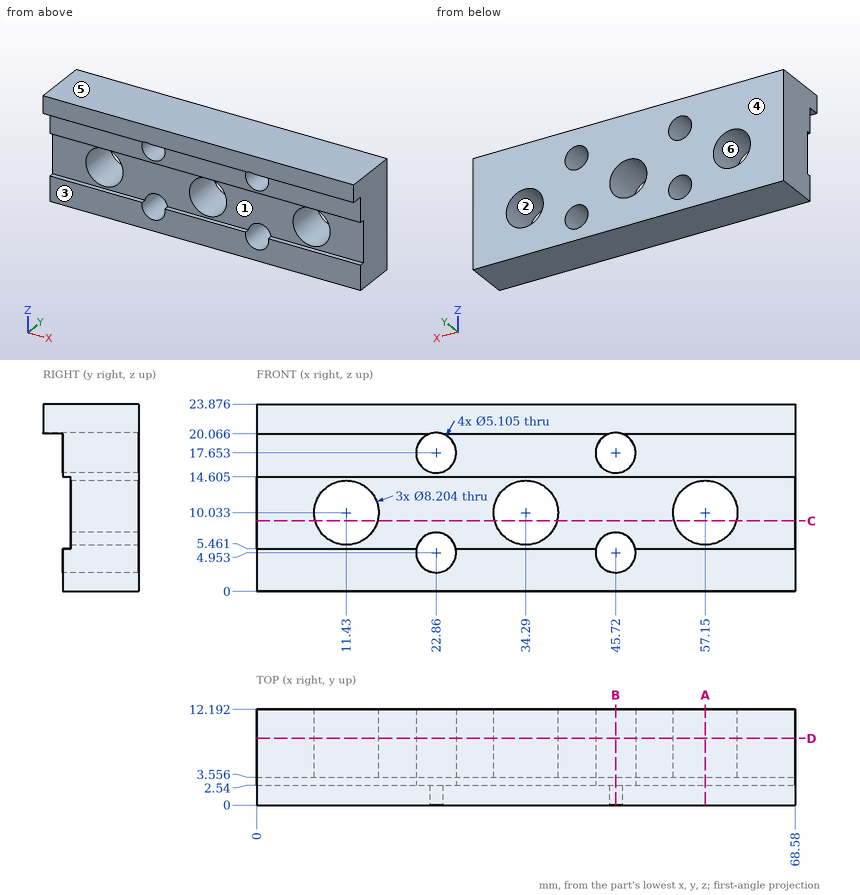
Design review of the part shown in the three views and the two pictorial views. Dimensions are in mm from the part's minimum x, y and z. A direction names the side the tool comes from. Round coordinates to 2 decimals unless told otherwise and drop trailing zeros. Write each loop counter-clockwise with the first axis right and the second up, starting at its lowest first coordinate (ties: lowest second). Pieces come first, ordered by that corner, then holes. Notation, with made-up numbers: (65.5, -2.5) - (92.5, -2.5) arc R34 ccw to (92.5, 27.5) - close; hole circle Ø9 at (47.25, 39.25). An arc over 180 degrees is marked (long way). Write item = value, one per line. Start each with the question number.
1. Consider section D-D on y = 8.5. Give the number of separate pieces and of enclosed holes in the cut face, plus the area to 3 significant figures.
2. Consider section C-C on z = 9. State the section outline as (x, y) points.
3. For pin 1 Ø5 at (y, z) = (2.5, 13) entering from -X; pin 2 Ø12 at (x, z) = (41, 9.5) entering from -Y, all flat-tipped, find the tip position at first contact; note any pin that passes through.
4. Wall thickness on L1, parallel to Z at x = 22.86, y = 9.5 (1 decimal); L2, parallel to Z at x = 45.5, y = 3.5 (1 decimal); L3, parallel to X at y = 6, z = 5: over which ranges is each line inside the solid? List them lowest first.
5. Draft analysis for pull direction Z (two halves, no side actions). For the marked faces 4, 5 and 6, state which applies: released by +Z, released by -Z, zero draft, split by the parting line, or undercut.
6. Consider section A-A on x = 57.15. State the section outline as (y, z) points (1 decimal), plus the area to 3 significant figures.
7. Consider section B-B on x = 45.72. State the section outline as (y, z) points (1 decimal), plus the area to 3 significant figures.
8. For the marked faces 1, 2 and 3, list the 3-axis set-ups (+Z, -Z, +X, -X, +Y, -Y) from which the entire face can be reached by the end or side of a thin tool; tool diameter is ignored.
Evaluation:
q1.separate_pieces = 1
q1.enclosed_holes = 7
q1.area = 1,400 mm2
q2.outline = (0, 3.56) - (7.46, 3.56) - (7.46, 12.19) - (0, 12.19) - close; (15.4, 3.56) - (30.32, 3.56) - (30.32, 12.19) - (15.4, 12.19) - close; (38.26, 3.56) - (53.18, 3.56) - (53.18, 12.19) - (38.26, 12.19) - close; (61.12, 3.56) - (68.58, 3.56) - (68.58, 12.19) - (61.12, 12.19) - close
q3.pin_1 = 0
q3.pin_2 = 2.54
q4.L1 = 0 to 2.4, 7.5 to 15.1, 20.2 to 23.9
q4.L2 = 0 to 2.4, 14.6 to 15.1, 20.2 to 23.9
q4.L3 = 0 to 20.31, 25.41 to 43.17, 48.27 to 68.58
q5.face_4 = zero draft
q5.face_5 = released by +Z
q5.face_6 = undercut
q6.outline = (0, 20.1) - (2.5, 20.1) - (2.5, 14.6) - (3.6, 14.6) - (3.6, 14.1) - (12.2, 14.1) - (12.2, 23.9) - (0, 23.9) - close; (2.5, 0) - (12.2, 0) - (12.2, 5.9) - (3.6, 5.9) - (3.6, 5.5) - (2.5, 5.5) - close
q6.area = 160 mm2
q7.outline = (0, 20.2) - (12.2, 20.2) - (12.2, 23.9) - (0, 23.9) - close; (2.5, 0) - (12.2, 0) - (12.2, 2.4) - (2.5, 2.4) - close; (2.5, 14.6) - (3.6, 14.6) - (3.6, 7.5) - (12.2, 7.5) - (12.2, 15.1) - (2.5, 15.1) - close
q7.area = 134 mm2
q8.face_1 = +X, -X, -Y
q8.face_2 = +Y, -Y
q8.face_3 = -Z, +X, -X, -Y
